```python
from build123d import *

# Parameters (mm, degrees)
CROQUIS1_W                        = 23
CROQUIS1_H                        = 48.2
SALIENTE_EXTRUIR1_DEPTH           = 22.5
VACIADO1_T                        = -4
CORTAR_EXTRUIR1_START             = -9.2
CORTAR_EXTRUIR1_DEPTH             = 3.5
REDONDEO1_R                       = 4
CROQUIS3_W                        = 11.8
CROQUIS3_H                        = 2.5
CORTAR_EXTRUIR2_DEPTH             = 23.5
CORTAR_EXTRUIR2_DEPTH_BACK        = 23.5
CORTAR_EXTRUIR3_REACH             = 50.2
CROQUIS4_R                        = 1
CORTAR_EXTRUIR3_DIRECTION_2_DEPTH = 1
CROQUIS5_R                        = 1
CORTAR_EXTRUIR4_DEPTH             = 5
SALIENTE_EXTRUIR2_REACH           = 25
CORTAR_EXTRUIR5_START             = -12
CORTAR_EXTRUIR5_DEPTH             = 13
SALIENTE_EXTRUIR3_REACH           = 25


with BuildPart() as part:
    # Croquis1 → Saliente-Extruir1 (new body, symmetric)
    with BuildSketch(Plane(origin=(0, 0, 0), x_dir=(0, 0, -1), z_dir=(1, 0, 0))):
        Rectangle(CROQUIS1_W, CROQUIS1_H)
    extrude(amount=SALIENTE_EXTRUIR1_DEPTH, both=True)

    # Vaciado1
    vaciado1_openings = [part.faces().sort_by_distance(p)[0] for p in [
        (0, 0, 11.5),
    ]]
    offset(amount=VACIADO1_T, openings=vaciado1_openings, kind=Kind.INTERSECTION)

    # Croquis2 → Cortar-Extruir1 (cut)
    with BuildSketch(Plane(origin=(0, 24.1, 0), x_dir=(1, 0, 0), z_dir=(0, 1, 0)).offset(CORTAR_EXTRUIR1_START)):
        Polygon((-22.5, 11.5), (-5.9, 11.5), (-5.9, 7.5), (-18.5, 7.5), (-18.5, 0), (-22.5, 0), align=None)
        Polygon((18.5, 0), (22.5, 0), (22.5, 11.5), (5.9, 11.5), (5.9, 7.5), (18.5, 7.5), align=None)
    extrude(amount=CORTAR_EXTRUIR1_DEPTH, mode=Mode.SUBTRACT)

    # Redondeo1
    redondeo1_edges = [part.edges().sort_by_distance(p)[0] for p in [
        (-22.5, 21.25, -11.5),
        (22.5, 21.25, -11.5),
        (22.5, -4.6, -11.5),
        (-22.5, -4.6, -11.5),
    ]]
    fillet(redondeo1_edges, radius=REDONDEO1_R)

    # Croquis3 → Cortar-Extruir2 (cut, two sides)
    with BuildSketch(Plane(origin=(0, 0, 0), x_dir=(0, 0, -1), z_dir=(1, 0, 0))) as cortar_extruir2_sk:
        with Locations((1.6, 3.35)):
            Rectangle(CROQUIS3_W, CROQUIS3_H)
    extrude(amount=CORTAR_EXTRUIR2_DEPTH, mode=Mode.SUBTRACT)
    extrude(cortar_extruir2_sk.sketch, amount=-CORTAR_EXTRUIR2_DEPTH_BACK, mode=Mode.SUBTRACT)

    # Croquis4 → Cortar-Extruir3 (cut, up to next)
    with BuildSketch(Plane(origin=(0, 24.1, 0), x_dir=(1, 0, 0), z_dir=(0, 1, 0)), mode=Mode.PRIVATE) as cortar_extruir3_sk1:
        Circle(CROQUIS4_R)
    cortar_extruir3_tool1 = extrude(cortar_extruir3_sk1.sketch, amount=-CORTAR_EXTRUIR3_REACH, mode=Mode.PRIVATE) & part.part
    add(cortar_extruir3_tool1.solids().sort_by_distance((0, 24.1, 0))[0], mode=Mode.SUBTRACT)

    # Croquis4 → Cortar-Extruir3 direction 2 (cut)
    with BuildSketch(Plane(origin=(0, 24.1, 0), x_dir=(1, 0, 0), z_dir=(0, 1, 0))):
        Circle(CROQUIS4_R)
    extrude(amount=CORTAR_EXTRUIR3_DIRECTION_2_DEPTH, mode=Mode.SUBTRACT)

    # Croquis5 → Cortar-Extruir4 (cut)
    with BuildSketch(Plane.XY.offset(11.5)):
        with Locations((0, 22.1)):
            Circle(CROQUIS5_R)
    extrude(amount=-CORTAR_EXTRUIR4_DEPTH, mode=Mode.SUBTRACT)

    # Croquis6 → Saliente-Extruir2 (add, up to next)
    with BuildSketch(Plane.XY.offset(11.5), mode=Mode.PRIVATE) as saliente_extruir2_sk1:
        with BuildLine():
            Line((-10, -20.1), (10, -20.1))
            ThreePointArc((10, -20.1), (8.271930009, -15.928069991), (4.1, -14.2))
            Line((4.1, -14.2), (-4.1, -14.2))
            ThreePointArc((-4.1, -14.2), (-8.271930009, -15.928069991), (-10, -20.1))
        make_face()
    saliente_extruir2_tool1 = extrude(saliente_extruir2_sk1.sketch, amount=-SALIENTE_EXTRUIR2_REACH, mode=Mode.PRIVATE) - part.part
    add(saliente_extruir2_tool1.solids().sort_by_distance((0, -17.386611, 11.5))[0])

    # Croquis7 → Cortar-Extruir5 (cut, through all)
    with BuildSketch(Plane(origin=(0, 24.1, 0), x_dir=(1, 0, 0), z_dir=(0, 1, 0)).offset(CORTAR_EXTRUIR5_START)):
        with BuildLine():
            Line((5.9, 7.5), (5.9, 0))
            Line((5.9, 0), (18.5, 0))
            Line((18.5, 0), (22.5, 0))
            Line((22.5, 0), (22.5, 7.5))
            ThreePointArc((22.5, 7.5), (21.328427125, 10.328427125), (18.5, 11.5))
            Line((18.5, 11.5), (5.9, 11.5))
            Line((5.9, 11.5), (5.9, 7.5))
        make_face()
    extrude(amount=CORTAR_EXTRUIR5_DEPTH, mode=Mode.SUBTRACT)

    # Croquis8 → Saliente-Extruir3 (add, up to next)
    with BuildSketch(Plane.XY.offset(11.5), mode=Mode.PRIVATE) as saliente_extruir3_sk1:
        with BuildLine():
            Line((-18.5, -20.1), (-18.5, 10.4))
            Line((-18.5, 10.4), (-10, 10.4))
            Line((-10, 10.4), (-10, -8.3))
            ThreePointArc((-10, -8.3), (-8.271930009, -12.471930009), (-4.1, -14.2))
            ThreePointArc((-4.1, -14.2), (-8.271930009, -15.928069991), (-10, -20.1))
            Line((-10, -20.1), (-18.5, -20.1))
        make_face()
    saliente_extruir3_tool1 = extrude(saliente_extruir3_sk1.sketch, amount=-SALIENTE_EXTRUIR3_REACH, mode=Mode.PRIVATE) - part.part
    add(saliente_extruir3_tool1.solids().sort_by_distance((-13.946608, -5.359479, 11.5))[0])


solid = part.part
```
For this review, take the finished solid that the model builds, in its own axes (mm). A direction names the side the tool comes from. Coordinates: 2 decimals unless noted, no trailing zeros. Write each loop counter-clockwise with the first axis right and the second up, starting at its lowest first coordinate (ties: lowest second). Pieces come first, ordered by that corner, then holes.
(1) Add section A-A on z = 8.75. Give the boundary of the cut face in (x, y).
(2) Wall thickness on probe 1 along Y at (x, z) = (0, 8.5); probe 2 along X at (y, z) = (1, -5); probe 3 along Y at (x, z) = (0, -3.75): over which ranges is each line inside the solid? List them lowest first.
(3) Add section D-D on y = 22.1. Give the boundary of the cut face in (x, z).
(4) The part is to be moulded in two halves that separate along Y. For faces 5 (the face through (-20, 3, -7.5)), 6 (the face through (20, 3, 4.3)), 7 (the face through (0, -24.1, 0)), 8 (the face through (21.359, -5.747, -10.297)), say which applies: +Y half, -Y half, draft (parallel to the pull), parting line (faces both ways), or undercut.
(5) Tool access review of faces 1 (the face through (20, 4.6, -2)), 2 (the face through (-14, 10.4, 2)), 3 (the face through (-5.9, 17, -10)), 4 (the face through (0, 22, 1)): name each direction out of +Z, -Z, +X, -X, +Y, -Y from which nothing blocks a thin tool from reaching the whole face with its end or side.
(6) Add section B-B on x = 0. Give the boundary of the cut face in (y, z).
(7) For pin 1 Ø1 at (y, z) = (17.5, -9.5) entering from -X; pin 2 Ø1.5 at (x, y) = (12, -12.5) entering from +Z; pin 3 Ø1 at (x, y) = (-21, 16) entering from -Z, all flat-tipped, find the tip position at first contact; note any pin that passes through.
(8) Add section C-C on z = -6.25. Give the boundary of the cut face in (x, y), then the cut area to 3 significant figures.
Answer sheet:
1. outline: (-22.5, -24.1) - (22.5, -24.1) - (22.5, 24.1) - (-22.5, 24.1) - close; hole (-18.5, 10.4) - (-10, 10.4) - (-10, -8.3) arc R5.9 ccw to (-4.1, -14.2) - (4.1, -14.2) arc R5.9 cw to (10, -20.1) - (18.5, -20.1) - (18.5, 20.1) - (-18.5, 20.1) - close; hole circle Ø2 at (0, 22.1)
2. probe 1: y = -24.1 to -14.2, 20.1 to 21.1, 23.1 to 24.1
2. probe 2: x = -22.5 to -10, 18.5 to 22.5
2. probe 3: y = -24.1 to -14.2, 20.1 to 24.1
3. outline: (-22.5, -7.5) arc R4 ccw to (-18.5, -11.5) - (5.9, -11.5) - (5.9, 0) - (22.5, 0) - (22.5, 11.5) - (1, 11.5) - (1, 6.5) - (-1, 6.5) - (-1, 11.5) - (-22.5, 11.5) - close; hole circle Ø2 at (0, 0)
4. face 5: undercut
4. face 6: undercut
4. face 7: -Y half
4. face 8: draft
5. face 1: +X
5. face 2: +Z
5. face 3: +Z, -Z, -X
5. face 4: +Y
6. outline: (-24.1, -11.5) - (24.1, -11.5) - (24.1, -1) - (20.1, -1) - (20.1, -7.5) - (-14.2, -7.5) - (-14.2, 11.5) - (-24.1, 11.5) - close; (20.1, 1) - (24.1, 1) - (24.1, 11.5) - (23.1, 11.5) - (23.1, 6.5) - (21.1, 6.5) - (21.1, 11.5) - (20.1, 11.5) - close
7. pin 1: stops at x = -5.9
7. pin 2: stops at z = -7.5
7. pin 3: stops at z = 0
8. outline: (-22.5, -24.1) - (22.5, -24.1) - (22.5, 2.1) - (18.5, 2.1) - (18.5, -20.1) - (10, -20.1) arc R5.9 ccw to (4.1, -14.2) - (-4.1, -14.2) arc R5.9 cw to (-10, -8.3) - (-10, 10.4) - (-18.5, 10.4) - (-18.5, 14.9) - (-22.5, 14.9) - (-22.5, 4.6) - (-18.5, 4.6) - (-18.5, 2.1) - (-22.5, 2.1) - close; (-22.5, 18.4) - (-18.5, 18.4) - (-18.5, 20.1) - (5.9, 20.1) - (5.9, 24.1) - (-22.5, 24.1) - close; (18.5, 4.6) - (22.5, 4.6) - (22.5, 12.1) - (18.5, 12.1) - close
8. area: 926 mm2
